Model file for the job. Use its own axes, mm. Face numbers are marked on the shaded views. A direction names the side the tool comes from. Round coordinates to 2 decimals unless told otherwise and drop trailing zeros. Loops run counter-clockwise (first coordinate to the right, second up) from the corner with the lowest first, then second, coordinate; pieces in that order, holes last. Notation, with made-up numbers: M 62.5,51 L 96.5,51 A32 cw 96.5,80 Z; hole C 82,39 d1. An arc over 180 degrees is marked long. Use a Markdown table: item, result. Add a question column.
Item 1: Saw through at A-A on x = 0.5. Write the cut outline in (y, z), then the cut area to 3 significant figures.
Item 2: Saw through at C-C on x = -5.13. Write the cut outline in (y, z) (3 decimals).
Item 3: Two-plate mould, pull along X, no slides. Class the marked faces 1, 2 and 3: +X half, -X half, draft (parallel to the pull), parting line (faces both ways), or undercut.
Item 4: Pin check, flat tips, straight feed: P1, Ø0.6, axis at x = 23.5, z = -19.5, coming from the -Y side; P2, Ø0.8, axis at x = -5, z = -19.5, coming from the +Y side. Stop position of each tip, or through.
Item 5: Saw through at B-B on y = 136. Write the cut outline in (x, z), then the cut area to 3 significant figures.
Item 6: Tool access for the marked faces 4, 5 and 6: list every direction of +Z, -Z, +X, -X, +Y, -Y with a clear straight run to the whole face (end or side of a thin tool).
Item 7: Wall check: L1, parallel to Z at x = 12.5, y = 132.25; L2, parallel to X at y = 133.75, z = -26.25; L3, parallel to X at y = 130.25, z = -18.25. Give the ranges that are in metal, low to high. Write a range as from..to.
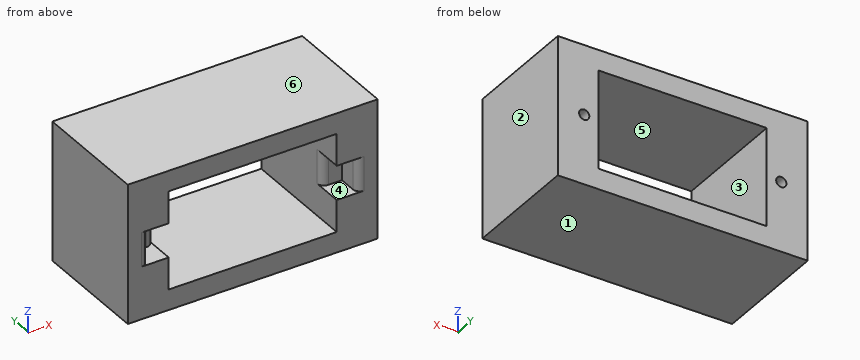
```python
from build123d import *

# Parameters (mm, degrees)
SKETCH040_W             = 36.6
SKETCH040_H             = 20.35
SKETCH040_W_2           = 24.6
SKETCH040_H_2           = 14.35
PAD021_DEPTH            = 17.31
SKETCH042_R             = 0.75
POCKET015_DEPTH         = 10
SKETCH041_W             = 3
SKETCH041_H             = 5
POCKET014_DEPTH         = 3.5
FILLET021_R             = 1
FILLET019_R             = 1
FILLET023_R             = 1
FILLET022_R             = 1
BODY010_PLACEMENT_ANGLE = 180


with BuildPart() as part:
    # Sketch040 (on Face1 of ReferencePocket006) → Pad021 (new body)
    with BuildSketch(Plane.XZ):
        with Locations((11.3, 6.175)):
            Rectangle(SKETCH040_W, SKETCH040_H)
        with Locations((11.3, 6.175)):
            Rectangle(SKETCH040_W_2, SKETCH040_H_2, mode=Mode.SUBTRACT)
    extrude(amount=-PAD021_DEPTH)

    # Sketch042 (on Face10 of Pad022) → Pocket015 (cut)
    with BuildSketch(Plane(origin=(0, 19.97, 0), x_dir=(-1, 0, 0), z_dir=(0, 1, 0))):
        with Locations((-25.73, 6.175)):
            Circle(SKETCH042_R)
        with Locations((3.13, 6.175)):
            Circle(SKETCH042_R)
    extrude(amount=-POCKET015_DEPTH, mode=Mode.SUBTRACT)

    # Sketch041 (on Face4 of Pocket015) → Pocket014 (cut)
    with BuildSketch(Plane.XZ):
        with Locations((-2.5, 6.175)):
            Rectangle(SKETCH041_W, SKETCH041_H)
        with Locations((25.1, 6.175)):
            Rectangle(SKETCH041_W, SKETCH041_H)
    extrude(amount=-POCKET014_DEPTH, mode=Mode.SUBTRACT)

    # Fillet021
    fillet021_edges = [part.edges().sort_by_distance(p)[0] for p in [
        (26.6, 0, 6.175),
    ]]
    fillet(fillet021_edges, radius=FILLET021_R)

    # Fillet019
    fillet019_edges = [part.edges().sort_by_distance(p)[0] for p in [
        (23.6, 3.5, 6.175),
    ]]
    fillet(fillet019_edges, radius=FILLET019_R)

    # Fillet023
    fillet023_edges = [part.edges().sort_by_distance(p)[0] for p in [
        (-1, 3.5, 6.175),
    ]]
    fillet(fillet023_edges, radius=FILLET023_R)

    # Fillet022
    fillet022_edges = [part.edges().sort_by_distance(p)[0] for p in [
        (-4, 0, 6.175),
    ]]
    fillet(fillet022_edges, radius=FILLET022_R)


with BuildPart() as part_1:
    # Body010 placement: moved
    add(part.part.moved(Location((20.600001, 126.400008, -13.43))).rotate(Axis((20.600001, 126.400008, -13.43), (0, 1, 0)), BODY010_PLACEMENT_ANGLE))


solid = part_1.part
```
Entries:
| question | item | result |
|---|---|---|
| 1 | outline | M 126.4,-29.78 L 143.71,-29.78 L 143.71,-26.78 L 126.4,-26.78 Z; M 126.4,-12.43 L 143.71,-12.43 L 143.71,-9.43 L 126.4,-9.43 Z |
| 1 | area | 104 mm2 |
| 2 | outline | M 126.4,-29.78 L 143.71,-29.78 L 143.71,-20.355 L 136.37,-20.355 L 136.37,-18.855 L 143.71,-18.855 L 143.71,-9.43 L 126.4,-9.43 L 126.4,-17.105 L 129.9,-17.105 L 129.9,-22.105 L 126.4,-22.105 Z |
| 3 | face 1 | draft |
| 3 | face 2 | +X half |
| 3 | face 3 | undercut |
| 4 | P1 | y = 129.9 |
| 4 | P2 | y = 136.37 |
| 5 | outline | M -9,-29.78 L 27.6,-29.78 L 27.6,-9.43 L -9,-9.43 Z; hole M -3,-26.78 L 21.6,-26.78 L 21.6,-12.43 L -3,-12.43 Z |
| 5 | area | 392 mm2 |
| 6 | face 4 | -Y |
| 6 | face 5 | +Y, -Y |
| 6 | face 6 | +Z, +X, -X, +Y, -Y |
| 7 | L1 | -29.78..-26.78, -12.43..-9.43 |
| 7 | L2 | -9..-3, 21.6..27.6 |
| 7 | L3 | -9..-3.24, 21.84..27.6 |
